Input: part model. Units: mm. Frame: model coordinates. A direction names the side the tool comes from. Give positions to 0.01 mm unless a question says otherwise; leave off trailing zeros. Order: outer loops, then holes, each group sorted by start corner. A loop starts at its lowest first (then second) coordinate and runs counter-clockwise, first axis right, second up. Notation, with made-up numbers: (-31.75, 43.5) - (-0.75, 43.5) arc R26 cw to (-0.75, 73.5) - close; hole circle Ø8 at (88.25, -3). An arc over 180 degrees is marked (long way). Answer in a Markdown table with one row per item. Add a question column.
1. Contact query for flat-ended pins moving along their axis: pin 1 (12 mm diameter, centred on x = -1, y = -6, fed in from +Z); pin 2 (3 mm diameter, centred on x = 15, y = -11, fed in from -Z); pin 3 (3 mm diameter, centred on y = 13, z = 501.5, fed in from -X) (3 decimals). Output: stop coordinate, or through.
2. Access query for faces 1 (the face through (-3, -15.875, 531)), 2 (the face through (19.05, 0, 531)). Directions: +Z, -Z, +X, -X, +Y, -Y. A direction counts if a zero-diameter tool reaches every point of the face in a straight line with its end or side. Return the directions, or none.
3. Ray query, line 1 (Y direction, x = -4, z = 590) (3 decimals); line 2 (X direction, y = 6, z = 497) (3 decimals); line 3 (X direction, y = -13, z = 555.5). Return the intervals inside material, ascending. Write a range as [from, to].
4. Mould query, pull axis Z, two halves, no side actions, for faces 3 (the face through (14.51, -14.44, 530.72)), 4 (the face through (13, -16, 449.6)), 5 (the face through (8, -17, 609.6)). Classes: released by +Z, released by -Z, zero draft, split by the parting line, or undercut.
5. Section query B-B on x = 0. Return loops of the section in (y, z) (3 decimals), and give its area (3 significant figures).
6. Section query C-C on y = -3.5. Return loops of the section in (x, z) (3 decimals).
```python
from build123d import *

# Parameters (mm, degrees)
BOSS_EXTRUDE1_DEPTH = 609.6
SKETCH3_W           = 635.2
SKETCH3_H           = 38.1
CUT_EXTRUDE1_DEPTH  = 60
SKETCH4_W           = 424
SKETCH4_H           = 38.1
CUT_EXTRUDE2_DEPTH  = 60


with BuildPart() as part:
    # Sketch2 → Boss-Extrude1 (new, symmetric)
    with BuildSketch(Plane.XY):
        with BuildLine():
            Line((-19.05, -19.05), (19.05, -19.05))
            Line((19.05, -19.05), (19.05, 19.05))
            Line((19.05, 19.05), (17.4625, 19.05))
            ThreePointArc((17.4625, 19.05), (16.339967985, 18.585032015), (15.875, 17.4625))
            Line((15.875, 17.4625), (15.875, -11.0998))
            ThreePointArc((15.875, -11.0998), (14.476376302, -14.476376302), (11.0998, -15.875))
            Line((11.0998, -15.875), (-17.4625, -15.875))
            ThreePointArc((-17.4625, -15.875), (-18.585032015, -16.339967985), (-19.05, -17.4625))
            Line((-19.05, -17.4625), (-19.05, -19.05))
        make_face()
    extrude(amount=BOSS_EXTRUDE1_DEPTH, both=True)

    # Sketch3 → Cut-Extrude1 (cut)
    with BuildSketch(Plane(origin=(19.05, 0, 0), x_dir=(0, 0, -1), z_dir=(1, 0, 0))):
        with Locations((292, 0)):
            Rectangle(SKETCH3_W, SKETCH3_H)
    extrude(amount=-CUT_EXTRUDE1_DEPTH, mode=Mode.SUBTRACT)

    # Sketch4 → Cut-Extrude2 (cut)
    with BuildSketch(Plane(origin=(19.05, 0, 0), x_dir=(0, 0, -1), z_dir=(1, 0, 0))):
        with Locations((-237.6, 0)):
            Rectangle(SKETCH4_W, SKETCH4_H)
    extrude(amount=-CUT_EXTRUDE2_DEPTH, mode=Mode.SUBTRACT)


solid = part.part
```
Answer:
| question | item | result |
|---|---|---|
| 1 | pin 1 | passes through |
| 1 | pin 2 | stops at z = 449.6 |
| 1 | pin 3 | stops at x = 15.875 |
| 2 | face 1 | +Z, -Z, -X, +Y |
| 2 | face 2 | +Z, -Z, +X, +Y, -Y |
| 3 | line 1 | y = [-19.05, -15.875] |
| 3 | line 2 | x = [15.875, 19.05] |
| 3 | line 3 | x = [15.48, 19.05] |
| 4 | face 3 | zero draft |
| 4 | face 4 | released by -Z |
| 4 | face 5 | released by +Z |
| 5 | outline | (-19.05, 449.6) - (-15.875, 449.6) - (-15.875, 609.6) - (-19.05, 609.6) - close |
| 5 | area | 508 mm² |
| 6 | outline | (15.875, 449.6) - (19.05, 449.6) - (19.05, 609.6) - (15.875, 609.6) - close |
